Geometry check sheet. Reference: the model listing, model coordinates, mm. Coordinates: 2 decimals unless noted, no trailing zeros. Loops run counter-clockwise (first coordinate to the right, second up) from the corner with the lowest first, then second, coordinate; pieces in that order, holes last.
from build123d import *

# Parameters (mm, degrees)
SKETCH2_W               = 160
SKETCH2_H               = 20
BOSS_EXTRUDE1_DEPTH     = 3.2
CUT_EXTRUDE1_DEPTH      = 162.276904732
CUT_EXTRUDE1_DEPTH_BACK = 162.276904732
SKETCH5_R               = 2
SKETCH6_R               = 1.5
CUT_EXTRUDE2_DEPTH      = 10
CUT_EXTRUDE3_DEPTH      = 162.276904732
CUT_EXTRUDE3_DEPTH_BACK = 162.276904732
SKETCH7_R               = 1
SKETCH8_R               = 1.5
CUT_EXTRUDE4_DEPTH      = 10


with BuildPart() as part:
    # Sketch2 → Boss-Extrude1 (new body)
    with BuildSketch(Plane(origin=(0, -10, 10), x_dir=(1, 0, 0), z_dir=(0, 0, -1))):
        with Locations((80, 0)):
            Rectangle(SKETCH2_W, SKETCH2_H)
    extrude(amount=BOSS_EXTRUDE1_DEPTH)

    # Sketch5 → Cut-Extrude1 (cut, two sides: drawn at the far end of the back side and taken through both)
    with BuildSketch(Plane.XY.offset(10).offset(-CUT_EXTRUDE1_DEPTH_BACK)):
        with Locations((131, -13)):
            Circle(SKETCH5_R)
        with Locations((29, -13)):
            Circle(SKETCH5_R)
    extrude(amount=CUT_EXTRUDE1_DEPTH + CUT_EXTRUDE1_DEPTH_BACK, mode=Mode.SUBTRACT)

    # Sketch6 → Cut-Extrude2 (cut)
    with BuildSketch(Plane.XY.offset(10)):
        with Locations((64, -9)):
            Circle(SKETCH6_R)
        with Locations((96, -9)):
            Circle(SKETCH6_R)
    extrude(amount=-CUT_EXTRUDE2_DEPTH, mode=Mode.SUBTRACT)

    # Sketch7 → Cut-Extrude3 (cut, two sides: drawn at the far end of the back side and taken through both)
    with BuildSketch(Plane.XY.offset(10).offset(-CUT_EXTRUDE3_DEPTH_BACK)):
        with Locations((3, -15)):
            Circle(SKETCH7_R)
        with Locations((3, -5)):
            Circle(SKETCH7_R)
    extrude(amount=CUT_EXTRUDE3_DEPTH + CUT_EXTRUDE3_DEPTH_BACK, mode=Mode.SUBTRACT)

    # Sketch8 → Cut-Extrude4 (cut)
    with BuildSketch(Plane.XY.offset(10)):
        with Locations((140, -13)):
            Circle(SKETCH8_R)
        with Locations((122, -13)):
            Circle(SKETCH8_R)
    extrude(amount=-CUT_EXTRUDE4_DEPTH, mode=Mode.SUBTRACT)


solid = part.part
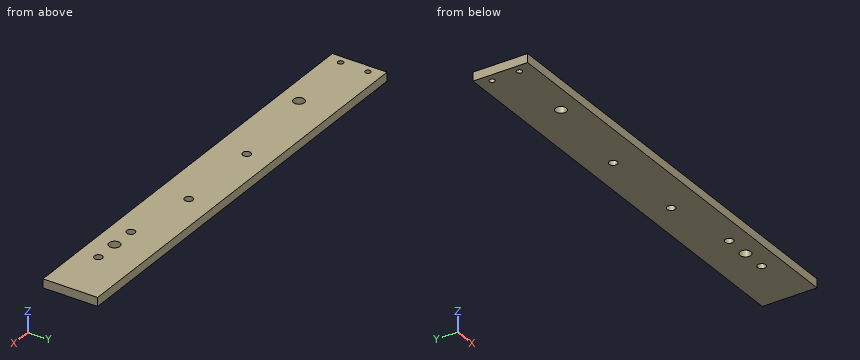
1) Material ranges on probe 1 along Y at (x, z) = (3, 8.35); probe 2 along Y at (x, z) = (131, 6.95); probe 3 along Y at (x, z) = (122, 7.8), recorded low to high.
Data:
probe 1: y = -20 to -16, -14 to -6, -4 to 0
probe 2: y = -20 to -15, -11 to 0
probe 3: y = -20 to -14.5, -11.5 to 0
2) Section check A-A on x = 64. Record the cut outline in (y, z).
Data:
outline: (-20, 6.8) - (-10.5, 6.8) - (-10.5, 10) - (-20, 10) - close; (-7.5, 6.8) - (0, 6.8) - (0, 10) - (-7.5, 10) - close
3) Section check C-C on x = 131. Record the cut outline in (y, z).
Data:
outline: (-20, 6.8) - (-15, 6.8) - (-15, 10) - (-20, 10) - close; (-11, 6.8) - (0, 6.8) - (0, 10) - (-11, 10) - close
4) Section check B-B on z = 7.95. Count the separate pieces of the cut face and the enclosed holes in it, and give its area (3 significant figures).
Data:
separate pieces: 1
enclosed holes: 8
area: 3,140 mm2
5) Depth check by flat-ended pin: pin 1 (1.2 mm diameter, centred on x = 3, y = -15, fed in from +Z). Enter the tip coordinate at first touch or a pass-through.
Data:
pin 1: passes through
